```python
from build123d import *

# Parameters (mm, degrees)
BOSS_EXTRUDE1_DEPTH   = 3.175
BOSS_EXTRUDE1_2_DEPTH = 3.175
SKETCH2_W             = 3.175
SKETCH2_H             = 36.35
BOSS_EXTRUDE2_DEPTH   = 3.175
SKETCH3_W             = 3.175
SKETCH3_H             = 3.175
BOSS_EXTRUDE8_DEPTH   = 423.175
BOSS_EXTRUDE8_2_DEPTH = 423.175
SKETCH4_W             = 3.175
SKETCH4_H             = 36.35
CUT_EXTRUDE1_DEPTH    = 427.326430831
CUT_EXTRUDE5_DEPTH    = 408.294257878
BOSS_EXTRUDE9_DEPTH   = 3.175
SKETCH8_R             = 22.246551504
CUT_EXTRUDE6_DEPTH    = 30
SKETCH9_W             = 3.175
SKETCH9_H             = 3.175
BOSS_EXTRUDE10_DEPTH  = 9.525
SKETCH10_W            = 3.036361865
SKETCH10_H            = 1.134211297
CUT_EXTRUDE7_DEPTH    = 10


with BuildPart() as part:
    # Sketch1 → Boss-Extrude1 (new body)
    with BuildSketch(Plane.XY):
        Polygon((15, 45), (405, 45), (405, 48.175), (18.175, 48.175), (-18.175, 48.175), (-18.175, 45), (-15, 45), align=None)
    extrude(amount=BOSS_EXTRUDE1_DEPTH)



with BuildPart() as body_2:
    # Sketch1 → Boss-Extrude1 2 (new body)
    with BuildSketch(Plane.XY):
        Polygon((-18.175, 15), (-15, 15), (15, 15), (405, 15), (405, 11.825), (18.175, 11.825), (-18.175, 11.825), align=None)
    extrude(amount=BOSS_EXTRUDE1_2_DEPTH)


with BuildPart() as part_1:
    add(part.part)

    add(body_2.part)  # Boss-Extrude2 merges body 2
    # Sketch2 → Boss-Extrude2 (add)
    with BuildSketch(Plane.XY.offset(3.175)):
        with Locations((-16.5875, 30)):
            Rectangle(SKETCH2_W, SKETCH2_H)
        Polygon((15, 11.825), (22.589723325, 11.825), (112.5, 46.473699254), (112.5, 12.285600704), (112.5, 11.825), (120.025102002, 11.825), (208.4125, 46.469905429), (208.4125, 11.825), (215.937602002, 11.825), (304.325, 46.469905429), (304.325, 11.825), (311.914723325, 11.825), (401.825, 46.473699254), (401.825, 11.825), (405, 11.825), (405, 48.175), (397.410276675, 48.175), (307.5, 13.526300746), (307.5, 48.175), (299.974897998, 48.175), (211.5875, 13.530094571), (211.5875, 48.175), (204.062397998, 48.175), (115.675, 13.530094571), (115.675, 48.175), (108.085276675, 48.175), (18.175, 13.526300746), (18.175, 48.175), (15, 48.175), align=None)
    extrude(amount=BOSS_EXTRUDE2_DEPTH)

    # Sketch4 → Cut-Extrude1 (cut, through all)
    with BuildSketch(Plane(origin=(405, 0, 0), x_dir=(0, 0, -1), z_dir=(1, 0, 0))):
        with Locations((-1.5875, 30)):
            Rectangle(SKETCH4_W, SKETCH4_H)
    extrude(amount=-CUT_EXTRUDE1_DEPTH, mode=Mode.SUBTRACT)


with BuildPart() as body_2_2:
    # Sketch3 → Boss-Extrude8 (new body)
    with BuildSketch(Plane(origin=(405, 0, 0), x_dir=(0, 0, -1), z_dir=(1, 0, 0))):
        with Locations((-4.7625, 49.7625)):
            Rectangle(SKETCH3_W, SKETCH3_H)
    extrude(amount=-BOSS_EXTRUDE8_DEPTH)


with BuildPart() as body_3:
    # Sketch3 → Boss-Extrude8 2 (new body)
    with BuildSketch(Plane(origin=(405, 0, 0), x_dir=(0, 0, -1), z_dir=(1, 0, 0))):
        with Locations((-4.7625, 10.2375)):
            Rectangle(SKETCH3_W, SKETCH3_H)
    extrude(amount=-BOSS_EXTRUDE8_2_DEPTH)


with BuildPart() as cut_extrude1_piece_1:
    # of the separate pieces the step leaves, piece 1, a body of its own (cut_extrude1_pieces)
    add(part_1.part.solids().sort_by_distance((401.825, 11.825, 3.175))[0])


with BuildPart() as cut_extrude1_piece_2:
    # of the separate pieces the step leaves, piece 2, a body of its own (cut_extrude1_pieces)
    add(part_1.part.solids().sort_by_distance((-15, 48.175, 3.175))[0])


with BuildPart() as cut_extrude5_tool:
    # Sketch5 → Cut-Extrude5 (new, through all)
    with BuildSketch(Plane.XZ.offset(-8.65)):
        Polygon((-18.175, 6.35), (-18.175, 3.175), (381.963638135, 3.175), (390.463332101, 6.35), align=None)
        Polygon((405, 6.35), (399.536667899, 6.35), (391.036973934, 3.175), (405, 3.175), align=None)
    extrude(amount=-CUT_EXTRUDE5_DEPTH)


with BuildPart() as body_2_2_1:
    add(body_2_2.part)

    # Cut-Extrude5: cut by cut_extrude5_tool
    add(cut_extrude5_tool.part, mode=Mode.SUBTRACT)


with BuildPart() as body_3_1:
    add(body_3.part)

    # Cut-Extrude5: cut by cut_extrude5_tool
    add(cut_extrude5_tool.part, mode=Mode.SUBTRACT)

    # Sketch5<3> → Boss-Extrude9 (add)
    with BuildSketch(Plane.XZ.offset(-8.65)):
        with BuildLine():
            Line((391.036973934, 3.175), (381.963638135, 3.175))
            Line((381.963638135, 3.175), (13.554929678, -134.441442909))
            ThreePointArc((13.554929678, -134.441442909), (14.260668904, -135.872458965), (14.665946091, -137.415710471))
            Line((14.665946091, -137.415710471), (391.036973934, 3.175))
        make_face()
        with BuildLine():
            ThreePointArc((14.665946091, -137.415710471), (14.260668904, -135.872458965), (13.554929678, -134.441442909))
            Line((13.554929678, -134.441442909), (9.243759355, -136.051849805))
            Line((9.243759355, -136.051849805), (10.354775769, -139.026117367))
            Line((10.354775769, -139.026117367), (14.665946091, -137.415710471))
        make_face()
    extrude(amount=-BOSS_EXTRUDE9_DEPTH)

    # Sketch9 → Boss-Extrude10 (add)
    with BuildSketch(Plane(origin=(-36.486342691, 0, -13.62921283), x_dir=(-0.34992642955188064, 0, 0.93677718476758), z_dir=(-0.93677718476758, 0, -0.34992642955188064))):
        with Locations((-132.27240455, 10.2375)):
            Rectangle(SKETCH9_W, SKETCH9_H)
    extrude(amount=BOSS_EXTRUDE10_DEPTH)

    # Sketch10 → Cut-Extrude7 (cut)
    with BuildSketch(Plane.XZ.offset(-8.65)):
        with Locations((398.018486967, 5.782894352)):
            Rectangle(SKETCH10_W, SKETCH10_H)
    extrude(amount=-CUT_EXTRUDE7_DEPTH, mode=Mode.SUBTRACT)


with BuildPart() as cut_extrude1_piece_1_1:
    add(cut_extrude1_piece_1.part)

    # Cut-Extrude5: cut by cut_extrude5_tool
    add(cut_extrude5_tool.part, mode=Mode.SUBTRACT)


with BuildPart() as cut_extrude1_piece_2_1:
    add(cut_extrude1_piece_2.part)

    # Cut-Extrude5: cut by cut_extrude5_tool
    add(cut_extrude5_tool.part, mode=Mode.SUBTRACT)


with BuildPart() as cut_extrude6_tool:
    # Sketch8 → Cut-Extrude6 (new body)
    with BuildSketch(Plane(origin=(0, 51.35, 0), x_dir=(1, 0, 0), z_dir=(0, 1, 0))):
        with Locations((390.031158892, -4.957539076)):
            Circle(SKETCH8_R)
    extrude(amount=-CUT_EXTRUDE6_DEPTH)


with BuildPart() as body_2_2_2:
    add(body_2_2_1.part)

    # Cut-Extrude6: cut by cut_extrude6_tool
    add(cut_extrude6_tool.part, mode=Mode.SUBTRACT)


with BuildPart() as cut_extrude1_piece_1_2:
    add(cut_extrude1_piece_1_1.part)

    # Cut-Extrude6: cut by cut_extrude6_tool
    add(cut_extrude6_tool.part, mode=Mode.SUBTRACT)


solid = body_3_1.part
```
For this review, take the finished solid that the model builds, in its own axes (mm). Coordinates: 2 decimals unless noted, no trailing zeros. Order: outer loops, then holes, each group sorted by start corner. A loop starts at its lowest first (then second) coordinate and runs counter-clockwise, first axis right, second up. Notation, with made-up numbers: (-35.5, 76) - (-26.5, 76) arc R21 cw to (-26.5, 113) - close; hole circle Ø3 at (-11.5, 43). An arc over 180 degrees is marked (long way). Answer as a JSON object with one key per item and string values. Group by question number.
1. We need section C-C on x = 124.5. State the section outline as (y, z) points (3 decimals).
2. We need section B-B on z = -46. State the section outline as (x, y) points (3 decimals).
3. Clearance check with a flat-ended pin moving along its axis: P1, Ø1, axis at x = 216.5, y = 10.5, coming from the -Z side. State where the tip first meets the part, or that it passes through.
4. For probe 1 along Z at (x, y) = (125.5, 9.75); probe 2 along Z at (x, y) = (80.5, 10.1), list the stretches that pass through material, from the lowest coordinate up.
5. We need section A-A on y = 11.15. State the section outline as (x, z) points (3 decimals), then the cut area to 3 significant figures.
Final values:
{
 "1": {"outline": "(8.65, -96.388) - (11.825, -96.388) - (11.825, -92.999) - (8.65, -92.999) - close"},
 "2": {"outline": "(250.319, 8.65) - (259.392, 8.65) - (259.392, 11.825) - (250.319, 11.825) - close"},
 "3": {"P1": "z = -62.21"},
 "4": {"probe 1": "-96.01 to -92.63", "probe 2": "-112.82 to -109.43"},
 "5": {"outline": "(0.321, -139.385) - (1.432, -142.359) - (396.5, 5.216) - (396.5, 6.35) - (390.463, 6.35) - close", "area": "1,330 mm²"}
}
